For this review, take the finished solid that the model builds, in its own axes (mm). A direction names the side the tool comes from. Round coordinates to 2 decimals unless told otherwise and drop trailing zeros. Order: outer loops, then holes, each group sorted by start corner. A loop starts at its lowest first (then second) coordinate and runs counter-clockwise, first axis right, second up. Notation, with made-up numbers: M 61.25,60 L 67.25,60 A24 cw 67.25,98 Z; hole C 50,24 d6. An arc over 180 degrees is marked long. Use a Markdown table: item, result.
from build123d import *
from OCP.BRepFilletAPI import BRepFilletAPI_MakeChamfer

# Parameters (mm, degrees)
CROQUIS1_W                 = 220.407444928
CROQUIS1_H                 = 139.358729484
CROQUIS1_W_2               = 180
CROQUIS1_H_2               = 113.81
SALIENTE_EXTRUIR1_DEPTH    = 2
EXTRUIR_L_MINA3_DEPTH      = 16.5
EXTRUIR_L_MINA3_DEPTH_BACK = 2
CROQUIS2_W                 = 226.407444928
CROQUIS2_H                 = 145.358729484
CROQUIS2_W_2               = 220.407444928
CROQUIS2_H_2               = 139.358729484
CROQUIS6_W                 = 222.447038553
CROQUIS6_H                 = 141.398323109
CORTAR_EXTRUIR2_DEPTH      = 16.5
CORTAR_EXTRUIR3_REACH      = 240.505
CORTAR_EXTRUIR4_DEPTH      = 1.960406375
REDONDEO2_R                = 0.7
CHAFL_N1_SIZE              = 1.5
CHAFL_N1_SIZE2             = 4.121216129
REDONDEO3_R                = 0.7


with BuildPart() as part:
    # Croquis1 → Saliente-Extruir1 (new body)
    with BuildSketch(Plane(origin=(0, 0, 0), x_dir=(1, 0, 0), z_dir=(0, 1, 0))):
        Rectangle(CROQUIS1_W, CROQUIS1_H)
        Rectangle(CROQUIS1_W_2, CROQUIS1_H_2, mode=Mode.SUBTRACT)
    extrude(amount=SALIENTE_EXTRUIR1_DEPTH)

    # Croquis2 → Extruir-Lámina3 (add, two sides: drawn at the far end of the back side and taken through both)
    with BuildSketch(Plane(origin=(0, 2, 0), x_dir=(1, 0, 0), z_dir=(0, 1, 0)).offset(-EXTRUIR_L_MINA3_DEPTH_BACK)):
        Rectangle(CROQUIS2_W, CROQUIS2_H)
        Rectangle(CROQUIS2_W_2, CROQUIS2_H_2, mode=Mode.SUBTRACT)
    extrude(amount=EXTRUIR_L_MINA3_DEPTH + EXTRUIR_L_MINA3_DEPTH_BACK)

    # Croquis6 → Cortar-Extruir2 (cut)
    with BuildSketch(Plane(origin=(0, 18.5, 0), x_dir=(1, 0, 0), z_dir=(0, 1, 0))):
        with Locations((-0.019796812, 0.019796812)):
            Rectangle(CROQUIS6_W, CROQUIS6_H)
    extrude(amount=-CORTAR_EXTRUIR2_DEPTH, mode=Mode.SUBTRACT)

    # Cortar-Extruir3: up to this face of the body (flat: up to its plane)
    cortar_extruir3_end = Plane(part.part.faces().sort_by_distance((113.203722464, 9.25, 0))[0])
    # Croquis7 → Cortar-Extruir3 (cut, up to the picked face)
    with BuildSketch(Plane.ZY.offset(113.203722464), mode=Mode.PRIVATE) as cortar_extruir3_sk1:
        Polygon((-72.679364742, 18.5), (-72.679364742, 17.034353119), (72.679364742, 2.5), (72.679364742, 18.5), align=None)
    cortar_extruir3_tool1 = split(extrude(cortar_extruir3_sk1.sketch, amount=-CORTAR_EXTRUIR3_REACH, mode=Mode.PRIVATE), bisect_by=cortar_extruir3_end, keep=Keep.BOTH, mode=Mode.PRIVATE)
    add(cortar_extruir3_tool1.solids().sort_by(Axis((-113.203722, 13.12567, 20.160481), (1, 0, 0)))[0], mode=Mode.SUBTRACT)

    # Croquis8 → Cortar-Extruir4 (cut)
    with BuildSketch(Plane(origin=(0, 0, -72.679364742), x_dir=(-1, 0, 0), z_dir=(0, 0, -1))):
        with BuildLine():
            Line((-33.703722464, 17.034353119), (-74.703722464, 17.034353119))
            Line((-74.703722464, 17.034353119), (-74.703722464, 9.034353119))
            ThreePointArc((-74.703722464, 9.034353119), (-74.264382636, 7.973692947), (-73.203722464, 7.534353119))
            Line((-73.203722464, 7.534353119), (-35.203722464, 7.534353119))
            ThreePointArc((-35.203722464, 7.534353119), (-34.143062292, 7.973692947), (-33.703722464, 9.034353119))
            Line((-33.703722464, 9.034353119), (-33.703722464, 17.034353119))
        make_face()
    extrude(amount=-CORTAR_EXTRUIR4_DEPTH, mode=Mode.SUBTRACT)

    # Redondeo2
    redondeo2_edges = [part.edges().sort_by_distance(p)[0] for p in [
        (33.703722464, 12.936343049, -70.718958367),
        (34.143062292, 7.973692947, -70.718958367),
        (54.203722464, 7.534353119, -70.718958367),
        (74.264382636, 7.973692947, -70.718958367),
        (74.703722464, 12.936343049, -70.718958367),
        (74.703722464, 13.034353119, -72.679364742),
        (74.264382636, 7.973692947, -72.679364742),
        (54.203722464, 7.534353119, -72.679364742),
        (34.143062292, 7.973692947, -72.679364742),
        (33.703722464, 13.034353119, -72.679364742),
    ]]
    fillet(redondeo2_edges, radius=REDONDEO2_R)

    # Chaflán1: one chamfer whose edges measure the first distance from different faces: ONE call of the kernel's chamfer builder (chamfer() names one face for all edges)
    chafl_n1_edges_1 = [part.edges().sort_by_distance(p)[0] for p in [
        (90, 0, 0),
    ]]
    chafl_n1_side_1 = [part.faces().sort_by_distance(p)[0] for p in [
        (90, 1, 0),
    ]]
    chafl_n1_edges_2 = [part.edges().sort_by_distance(p)[0] for p in [
        (0, 0, -56.905),
    ]]
    chafl_n1_side_2 = [part.faces().sort_by_distance(p)[0] for p in [
        (0, 1, -56.905),
    ]]
    chafl_n1_edges_3 = [part.edges().sort_by_distance(p)[0] for p in [
        (-90, 0, 0),
    ]]
    chafl_n1_side_3 = [part.faces().sort_by_distance(p)[0] for p in [
        (-90, 1, 0),
    ]]
    chafl_n1_edges_4 = [part.edges().sort_by_distance(p)[0] for p in [
        (0, 0, 56.905),
    ]]
    chafl_n1_side_4 = [part.faces().sort_by_distance(p)[0] for p in [
        (0, 1, 56.905),
    ]]
    chafl_n1 = BRepFilletAPI_MakeChamfer(part.part.solid().wrapped)
    for e in chafl_n1_edges_1:
        chafl_n1.Add(CHAFL_N1_SIZE, CHAFL_N1_SIZE2, e.wrapped, chafl_n1_side_1[0].wrapped)  # the first distance lies on this face
    for e in chafl_n1_edges_2:
        chafl_n1.Add(CHAFL_N1_SIZE, CHAFL_N1_SIZE2, e.wrapped, chafl_n1_side_2[0].wrapped)  # the first distance lies on this face
    for e in chafl_n1_edges_3:
        chafl_n1.Add(CHAFL_N1_SIZE, CHAFL_N1_SIZE2, e.wrapped, chafl_n1_side_3[0].wrapped)  # the first distance lies on this face
    for e in chafl_n1_edges_4:
        chafl_n1.Add(CHAFL_N1_SIZE, CHAFL_N1_SIZE2, e.wrapped, chafl_n1_side_4[0].wrapped)  # the first distance lies on this face
    add(Compound.cast(chafl_n1.Shape()), mode=Mode.REPLACE)

    # Redondeo3
    redondeo3_edges = [part.edges().sort_by_distance(p)[0] for p in [
        (-113.203722464, 0, 0),
        (0, 0, -72.679364742),
        (113.203722464, 0, 0),
        (0, 0, 72.679364742),
    ]]
    fillet(redondeo3_edges, radius=REDONDEO3_R)

    # Partir1
    split(bisect_by=Plane(origin=(0, 0, 0), x_dir=(0, 0, 1), z_dir=(1, 0, 0)), keep=Keep.BOTTOM)


solid = part.part
Q1. Add section A-A (x = -39.5). Write out the cut boundary in (y, z) (3 decimals), then the cut area to 3 significant figures.
Determined:
| item | result |
|---|---|
| outline | M 0,-71.979 A0.7 ccw 0.7,-72.679 L 17.034,-72.679 L 16.838,-70.719 L 2,-70.719 L 2,-56.905 L 1.5,-56.905 L 0,-61.026 Z; M 0,61.026 L 1.5,56.905 L 2,56.905 L 2,70.679 L 2.7,70.679 L 2.5,72.679 L 0.7,72.679 A0.7 ccw 0,71.979 Z |
| area | 87.2 mm^2 |
Q2. Add section D-D (z = -25.5). Write out the cut boundary in (x, y).
Determined:
| item | result |
|---|---|
| outline | M -113.2,0.7 A0.7 ccw -112.5,0 L -94.12,0 L -90,1.5 L -90,2 L -111.24,2 L -111.24,12.32 L -113.2,12.32 Z |
Q3. Wall thickness on line 1 along Z through (x, y) = (-28, 1.75) (3 decimals); line 2 along Z through (x, y) = (-77, 13.5); line 3 along Y through (x, z) = (-88.5, 63): over which ranges is each line inside the solid? List them lowest first. Write a range as [from, to].
Determined:
| item | result |
|---|---|
| line 1 | z = [-72.679, -56.905], [56.905, 72.679] |
| line 2 | z = [-72.68, -70.72] |
| line 3 | y = [0, 2] |
Q4. Add section B-B (z = 34). Write out the cut boundary in (x, y), then the cut area to 3 significant figures.
Determined:
| item | result |
|---|---|
| outline | M -113.2,0.7 A0.7 ccw -112.5,0 L -94.12,0 L -90,1.5 L -90,2 L -111.24,2 L -111.24,6.37 L -113.2,6.37 Z |
| area | 51.8 mm^2 |
Q5. Machinability: for faces 1 (the flat face through (-47.72, 0.74, -58.99)), 2 (the flat face through (-113.204, 7, -15)), which of the approach directions +Z, -Z, +X, -X, +Y, -Y give a long, thin tool a straight path to every point of the face, cutting with its end or side? Answer none if there is none.
Determined:
| item | result |
|---|---|
| face 1 | +X, -Y |
| face 2 | +Z, -Z, -X, +Y, -Y |
Q6. Clearance check with flat-ended pins moving along their axes: pin 1 (8 mm diameter, centred on y = 9.5, z = 2, fed in from +X); pin 2 (12 mm diameter, centred on x = -87.5, z = -4.5, fed in from -Y); pin 3 (8 mm diameter, centred on x = -69.5, y = 7.5, fed in from +Z). State where each tip first meets the part, or that it passes through.
Determined:
| item | result |
|---|---|
| pin 1 | stops at x = -111.24 |
| pin 2 | stops at y = 0.23 |
| pin 3 | stops at z = -70.72 |
Q7. Add section C-C (y = 7.75). Write out the cut boundary in (x, z).
Determined:
| item | result |
|---|---|
| outline | M -113.2,-72.68 L 0,-72.68 L 0,-70.72 L -111.24,-70.72 L -111.24,20.17 L -113.2,20.17 Z |
Q8. Draft analysis for pull direction Z (two halves, no side actions). For faces 3 (the flat face through (-57, 9, -72.679)), 4 (the flat face through (0, 5, -71)), 5 (the flat face through (-93, 2, -1)), 6 (the flat face through (-47.72, 0.74, 58.99)), state which applies: pulls with the +Z half, pulls with the -Z half, needs draft (parallel to the pull), parting line crosses it, or undercut.
Determined:
| item | result |
|---|---|
| face 3 | pulls with the -Z half |
| face 4 | needs draft |
| face 5 | undercut |
| face 6 | undercut |
